from build123d import *

# Parameters (mm, degrees)
BOSS_EXTRUDE1_DEPTH               = 2
TAP_DRILL_FOR_M3_TAP1_D           = 2.5
TAP_DRILL_FOR_M3_TAP1_CSINK_D     = 2.55
TAP_DRILL_FOR_M3_TAP1_CSINK_ANGLE = 90


with BuildPart() as part:
    # Model → Boss-Extrude1 (new body)
    with BuildSketch(Plane.XY):
        with BuildLine():
            Line((-38, 14), (-38, -14))
            ThreePointArc((-38, -14), (-37.414213562, -15.414213562), (-36, -16))
            Line((-36, -16), (36, -16))
            ThreePointArc((36, -16), (37.414213562, -15.414213562), (38, -14))
            Line((38, -14), (38, 14))
            ThreePointArc((38, 14), (37.414213562, 15.414213562), (36, 16))
            Line((36, 16), (-36, 16))
            ThreePointArc((-36, 16), (-37.414213562, 15.414213562), (-38, 14))
        make_face()
    extrude(amount=BOSS_EXTRUDE1_DEPTH)

    # Tap Drill for M3 Tap1 (through all)
    with Locations(Plane.XY.offset(2)):
        with Locations((-33.5, 11.5), (-5.5, -11), (33.5, 11.5)):
            CounterSinkHole(TAP_DRILL_FOR_M3_TAP1_D / 2, TAP_DRILL_FOR_M3_TAP1_CSINK_D / 2, counter_sink_angle=TAP_DRILL_FOR_M3_TAP1_CSINK_ANGLE)


solid = part.part
Geometry check sheet. Reference: the model listing, model coordinates, mm. Give positions to 0.01 mm unless a question says otherwise; leave off trailing zeros. Order: outer loops, then holes, each group sorted by start corner. A loop starts at its lowest first (then second) coordinate and runs counter-clockwise, first axis right, second up. Notation, with made-up numbers: M -32.5,5 L 7.5,5 A31 ccw 7.5,31 Z; hole C 12,24.25 d6. An arc over 180 degrees is marked long. Use a Markdown table: item, result.
Item 1: Material ranges on line 1 along X through (y, z) = (-11, 0.5); line 2 along Y through (x, z) = (-5.5, 0.5); line 3 along Y through (x, z) = (-33.5, 1.3), recorded low to high.
Answers follow:
| item | result |
|---|---|
| line 1 | x = -38 to -6.75, -4.25 to 38 |
| line 2 | y = -16 to -12.25, -9.75 to 16 |
| line 3 | y = -16 to 10.25, 12.75 to 16 |
Item 2: Section check C-C (x = 33.5). Record the cut outline in (y, z) (3 decimals).
Answers follow:
| item | result |
|---|---|
| outline | M -16,0 L 10.25,0 L 10.25,1.975 L 10.225,2 L -16,2 Z; M 12.75,0 L 16,0 L 16,2 L 12.775,2 L 12.75,1.975 Z |
Item 3: Section check B-B (y = 11.5). Record the cut outline in (x, z) (3 decimals).
Answers follow:
| item | result |
|---|---|
| outline | M -38,0 L -34.75,0 L -34.75,1.975 L -34.775,2 L -38,2 Z; M -32.25,0 L 32.25,0 L 32.25,1.975 L 32.225,2 L -32.225,2 L -32.25,1.975 Z; M 34.75,0 L 38,0 L 38,2 L 34.775,2 L 34.75,1.975 Z |
Item 4: Draft check along X on faces 1 (the cylindrical face through (-37.4, 15.43, 0.99)), 2 (the cylindrical face through (37.43, 15.4, 0.99)), 3 (the cylindrical face through (-5.34, -9.76, 0.97)), 4 (the cylindrical face through (32.828, 12.554, 0.974)). Enter one of: +X half, -X half, draft (parallel to the pull), parting line (faces both ways), or undercut.
Answers follow:
| item | result |
|---|---|
| face 1 | -X half |
| face 2 | +X half |
| face 3 | undercut |
| face 4 | undercut |
Item 5: Depth check by flat-ended pin: P1, Ø3, axis at x = -33.5, y = 11.5, coming from the +Z side; P2, Ø2, axis at x = -5.5, y = -11, coming from the +Z side. Enter the tip coordinate at first touch or a pass-through.
Answers follow:
| item | result |
|---|---|
| P1 | stops at z = 2 |
| P2 | passes through |
Item 6: Section check A-A (y = -11). Record the cut outline in (x, z) (3 decimals).
Answers follow:
| item | result |
|---|---|
| outline | M -38,0 L -6.75,0 L -6.75,1.975 L -6.775,2 L -38,2 Z; M -4.25,0 L 38,0 L 38,2 L -4.225,2 L -4.25,1.975 Z |
